Input: part model. Units: mm. Frame: model coordinates. A direction names the side the tool comes from. Coordinates: 2 decimals unless noted, no trailing zeros. Order: outer loops, then holes, each group sorted by start corner. A loop starts at its lowest first (then second) coordinate and runs counter-clockwise, first axis right, second up. Notation, with made-up numbers: (64.25, -9) -> (95.25, -9) arc R23 cw to (95.25, 23) -> close; hole circle Ø7 at (6, -13). An arc over 180 degrees is marked (long way). One line per item, written item: value. Start each with the question number.
from build123d import *

# Parameters (mm, degrees)
BOSS_EXTRUDE1_DEPTH = 8
SKETCH4_W           = 10.258234738
SKETCH4_H           = 27
CUT_EXTRUDE1_DEPTH  = 3


with BuildPart() as part:
    # Sketch1 → Boss-Extrude1 (new body)
    with BuildSketch(Plane(origin=(0, 0, 0), x_dir=(1, 0, 0), z_dir=(0, 1, 0))):
        Polygon((-113, -12.62891462), (113, -12.62891462), (128.588457268, 14.37108538), (-128.588457268, 14.37108538), align=None)
    extrude(amount=BOSS_EXTRUDE1_DEPTH)

    # Sketch4 → Cut-Extrude1 (cut)
    with BuildSketch(Plane(origin=(0, 8, 0), x_dir=(1, 0, 0), z_dir=(0, 1, 0))):
        with Locations((-66, 0.87108538)):
            Rectangle(SKETCH4_W, SKETCH4_H)
        with Locations((-99, 0.87108538)):
            Rectangle(SKETCH4_W, SKETCH4_H)
        with Locations((-33, 0.87108538)):
            Rectangle(SKETCH4_W, SKETCH4_H)
        with Locations((0, 0.87108538)):
            Rectangle(SKETCH4_W, SKETCH4_H)
        with Locations((33, 0.87108538)):
            Rectangle(SKETCH4_W, SKETCH4_H)
        with Locations((66, 0.87108538)):
            Rectangle(SKETCH4_W, SKETCH4_H)
        with Locations((99, 0.87108538)):
            Rectangle(SKETCH4_W, SKETCH4_H)
    extrude(amount=-CUT_EXTRUDE1_DEPTH, mode=Mode.SUBTRACT)


solid = part.part
1) Ray query, line 1 along Y through (x, z) = (-96, 7.5); line 2 along X through (y, z) = (1.75, 10); line 3 along X through (y, z) = (2.5, -6.25). Return the intervals inside material, ascending. Write a range as from..to.
2) Mould query, pull axis X, two halves, no side actions, for faces 3 (the flat face through (33, 5, -1)), 4 (the flat face through (-120.903, 3.944, -1.06)), 5 (the flat face through (-50, 8, -1)), 6 (the flat face through (-66, 5, -1)). Classes: +X half, -X half, draft (parallel to the pull), parting line (faces both ways), or undercut.
3) Pin query (flat end, axial travel): pin 1 Ø3.5 at (y, z) = (6, 0.5) entering from +X; pin 2 Ø2.5 at (y, z) = (6.5, 3) entering from -X; pin 3 Ø3.5 at (y, z) = (6.5, 4.5) entering from +X. Return the tip coordinate at first contact, or that it passes through.
4) Access query for faces 1 (the flat face through (-17, 8, -1)), 2 (the flat face through (-33, 5, -1)). Directions: +Z, -Z, +X, -X, +Y, -Y. A direction counts if a zero-diameter tool reaches every point of the face in a straight line with its end or side. Return the directions, or none.
5) Section query C-C, the plane y = 2.25. Return the cut outline in (x, z).
6) Section query B-B, the plane x = -68.5. Return the cut outline in (y, z), plus the area to 3 significant figures.
Entries:
1. line 1: y = 0..5
1. line 2: x = -114.52..114.52
1. line 3: x = -123.9..123.9
2. face 3: undercut
2. face 4: -X half
2. face 5: draft
2. face 6: undercut
3. pin 1: stops at x = 121.01
3. pin 2: stops at x = -119.28
3. pin 3: stops at x = 118.7
4. face 1: +Z, -Z, +X, -X, +Y
4. face 2: +Z, -Z, +Y
5. outline: (-128.59, -14.37) -> (128.59, -14.37) -> (113, 12.63) -> (-113, 12.63) -> close
6. outline: (0, -14.37) -> (5, -14.37) -> (5, 12.63) -> (0, 12.63) -> close
6. area: 135 mm2
